Build history of the part. All positions in model axes, mm. A direction names the side the tool comes from. Give positions to 0.01 mm unless a question says otherwise; leave off trailing zeros. Order: outer loops, then holes, each group sorted by start corner. A loop starts at its lowest first (then second) coordinate and runs counter-clockwise, first axis right, second up. Notation, with made-up numbers: M 2,6.25 L 10,6.25 A11 cw 10,17.25 Z; hole C 40.25,30.25 d6. An arc over 180 degrees is marked long. One line per item, written item: value.
from build123d import *

# Parameters (mm, degrees)
BOTTOMEXTRUDE_DEPTH = 80
SHELL1_T            = -8
SKETCH3_W           = 102
SKETCH3_H           = 72
CUT_EXTRUDE1_DEPTH  = 160.70597985
SKETCH4_R           = 2.25
CUT_EXTRUDE2_DEPTH  = 6
SKETCH5_R           = 2.25
CUT_EXTRUDE3_DEPTH  = 6
FILLET2_R           = 2
FILLET3_R           = 2


with BuildPart() as part:
    # Sketch2 → BottomExtrude (new body)
    with BuildSketch(Plane(origin=(0, 0, 0), x_dir=(1, 0, 0), z_dir=(0, 1, 0))):
        with BuildLine():
            Line((-125, 59), (0, 59))
            ThreePointArc((0, 59), (59, 0), (0, -59))
            Line((0, -59), (-125, -59))
            Line((-125, -59), (-125, 59))
        make_face()
    extrude(amount=BOTTOMEXTRUDE_DEPTH)

    # Shell1
    shell1_openings = [part.faces().sort_by_distance(p)[0] for p in [
        (-38.824706597, 80, 0),
    ]]
    offset(amount=SHELL1_T, openings=shell1_openings, kind=Kind.INTERSECTION)

    # Sketch3 → Cut-Extrude1 (cut, through all)
    with BuildSketch(Plane(origin=(0, 0, 0), x_dir=(0, 0, -1), z_dir=(1, 0, 0))):
        with Locations((0, 44)):
            Rectangle(SKETCH3_W, SKETCH3_H)
    extrude(amount=-CUT_EXTRUDE1_DEPTH, mode=Mode.SUBTRACT)

    # Sketch4 → Cut-Extrude2 (cut)
    with BuildSketch(Plane.ZY.offset(125)):
        with Locations((-55, 70)):
            Circle(SKETCH4_R)
        with Locations((55, 70)):
            Circle(SKETCH4_R)
        with Locations((55, 5)):
            Circle(SKETCH4_R)
        with Locations((-55, 5)):
            Circle(SKETCH4_R)
    extrude(amount=-CUT_EXTRUDE2_DEPTH, mode=Mode.SUBTRACT)

    # Sketch5 → Cut-Extrude3 (cut)
    with BuildSketch(Plane(origin=(0, 80, 0), x_dir=(1, 0, 0), z_dir=(0, 1, 0))):
        with Locations(Location((0, 55, 0), (0, 0, 270))):
            Circle(SKETCH5_R)
        with Locations(Location((-110, 55, 0), (0, 0, 270))):
            Circle(SKETCH5_R)
        with Locations(Location((-110, -55, 0), (0, 0, 270))):
            Circle(SKETCH5_R)
        with Locations(Location((0, -55, 0), (0, 0, 270))):
            Circle(SKETCH5_R)
    extrude(amount=-CUT_EXTRUDE3_DEPTH, mode=Mode.SUBTRACT)

    # Fillet2
    # the kernel refuses this fillet: 2 mm, written as the material it takes off along each edge
    with BuildSketch(Plane(origin=(-125, -5, -59), x_dir=(0, 0, 1), z_dir=(0, 1, 0))) as fillet2_piece_1:
        with BuildLine():
            CenterArc((FILLET2_R, FILLET2_R), FILLET2_R, 180, 90)
            Line((0, FILLET2_R), (0, 0))
            Line((0, 0), (FILLET2_R, 0))
        make_face()
    extrude(amount=90, mode=Mode.SUBTRACT)

    # Fillet3
    # the kernel refuses this fillet: 2 mm, written as the material it takes off along each edge
    with BuildSketch(Plane(origin=(-125, -5, 59), x_dir=(1, 0, 0), z_dir=(0, 1, 0))) as fillet3_piece_1:
        with BuildLine():
            CenterArc((FILLET3_R, FILLET3_R), FILLET3_R, 180, 90)
            Line((0, FILLET3_R), (0, 0))
            Line((0, 0), (FILLET3_R, 0))
        make_face()
    extrude(amount=90, mode=Mode.SUBTRACT)


solid = part.part
1) Saw through at C-C, the plane z = 3.5. Write the cut outline in (x, y), then the cut area to 3 significant figures.
Check values:
outline: M -125,0 L 58.9,0 L 58.9,80 L 50.88,80 L 50.88,8 L -125,8 Z
area: 2,050 mm^2
2) Saw through at B-B, the plane x = -33. Write the cut outline in (y, z).
Check values:
outline: M 0,-59 L 80,-59 L 80,-51 L 8,-51 L 8,51 L 80,51 L 80,59 L 0,59 Z
3) Tool access for faces 1 (the face through (-36, 8, 1)), 2 (the face through (-119, 70, 55)), 3 (the face through (-125, 7, 0)), 4 (the face through (-112.196, 77.042, 54.512)): list every direction of +Z, -Z, +X, -X, +Y, -Y with a clear straight run to the whole face (end or side of a thin tool).
Check values:
face 1: -X, +Y
face 2: -X
face 3: +Z, -Z, -X, +Y, -Y
face 4: +Y
4) Drill centre lines: probe 1 along Y at (x, z) = (-121.5, -55); probe 2 along Z at (x, y) = (-122.25, 70); probe 3 along Z at (x, y) = (-123, 5). Where is each one in solid material? Low to high. Write a range as from..to.
Check values:
probe 1: 0..2.75, 7.25..67.75, 72.25..80
probe 2: -59..-57.25, -52.75..-51, 51..52.75, 57.25..59
probe 3: -59..-57.25, -52.75..52.75, 57.25..59
5) Saw through at A-A, the plane y = 40. Write the cut outline in (x, z).
Check values:
outline: M -125,-57 A2 ccw -123,-59 L 0,-59 A59 ccw 0,59 L -123,59 A2 ccw -125,57 L -125,51 L 0,51 A51 cw 0,-51 L -125,-51 Z
6) Pin check, flat tips, straight feed: pin 1 (2 mm diameter, centred on y = 69, z = -54.5, fed in from -X); pin 2 (4 mm diameter, centred on x = -8.5, z = 39.5, fed in from +Y); pin 3 (10 mm diameter, centred on y = 22.5, z = 41.5, fed in from -X). Stop position of each tip, or through.
Check values:
pin 1: x = -119
pin 2: y = 8
pin 3: x = 20.95
7) Mould opens along X. For faces 5 (the face through (-62, 43, 51)), 6 (the face through (0, 74, -55)), 7 (the face through (50.988, 43.496, -1.121)), 8 (the face through (0, 74, 55)) say: released by +X, released by -X, zero draft, split by the parting line, or undercut.
Check values:
face 5: zero draft
face 6: undercut
face 7: released by -X
face 8: undercut
8) Saw through at D-D, the plane x = -110. Write the cut outline in (y, z), then the cut area to 3 significant figures.
Check values:
outline: M 0,-59 L 80,-59 L 80,-57.25 L 74,-57.25 L 74,-52.75 L 80,-52.75 L 80,-51 L 8,-51 L 8,51 L 80,51 L 80,52.75 L 74,52.75 L 74,57.25 L 80,57.25 L 80,59 L 0,59 Z
area: 2,040 mm^2
